Verification items for the finished model (mm, model axes). Round coordinates to 2 decimals unless told otherwise and drop trailing zeros. Loops run counter-clockwise (first coordinate to the right, second up) from the corner with the lowest first, then second, coordinate; pieces in that order, holes last. Notation, with made-up numbers: (-32, 47.5) -> (24, 47.5) arc R17 cw to (24, 51.5) -> close; hole circle Ø3 at (26, 84). An arc over 180 degrees is marked (long way). Write item = value, one per line.
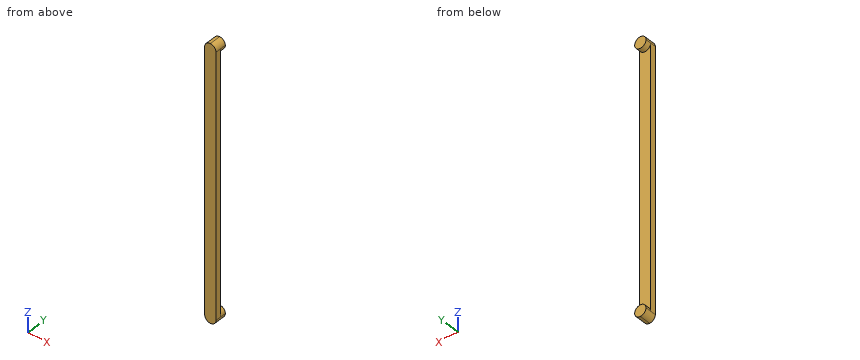
```python
from build123d import *

# Parameters (mm, degrees)
F1_DEPTH = 25.4
F2_DEPTH = 50.8


with BuildPart() as f1:
    # F0 (on Front) → F1 (new body)
    with BuildSketch(Plane.XZ):
        with BuildLine():
            Line((25.4, -584.2), (25.4, 584.2))
            ThreePointArc((25.4, 584.2), (0, 558.8), (-25.4, 584.2))
            Line((-25.4, 584.2), (-25.4, -584.2000000301))
            ThreePointArc((-25.4, -584.2000000301), (-1.51e-08, -558.8), (25.4, -584.2))
        make_face()
    extrude(amount=-F1_DEPTH)

    # F0 (on Front) → F2 (join)
    with BuildSketch(Plane.XZ):
        with BuildLine():
            ThreePointArc((25.4, 584.2), (17.9605121413, 602.160512343), (-2.853e-07, 609.6))
            ThreePointArc((-2.853e-07, 609.6), (-17.960512343, 602.1605121413), (-25.4, 584.2))
            ThreePointArc((-25.4, 584.2), (0, 558.8), (25.4, 584.2))
        make_face()
        with BuildLine():
            ThreePointArc((4.74e-07, -609.6), (17.9605124097, -602.1605120745), (25.4, -584.2))
            ThreePointArc((25.4, -584.2), (-1.51e-08, -558.8), (-25.4, -584.2000000301))
            ThreePointArc((-25.4, -584.2000000301), (-17.9605120639, -602.1605124204), (4.74e-07, -609.6))
        make_face()
    extrude(amount=-F2_DEPTH)


solid = f1.part
```
(1) Sectioned sample at A-A, the plane y = 34.5. Record the cut outline in (x, z).
Filled sheet:
outline = circle Ø50.8 at (0, -584.2); circle Ø50.8 at (0, 584.2)
(2) Sectioned sample at C-C, the plane z = 242.5. Record the cut outline in (x, y).
Filled sheet:
outline = (-25.4, 0) -> (25.4, 0) -> (25.4, 25.4) -> (-25.4, 25.4) -> close
(3) Go/stop test with flat-tipped pins: pin 1 Ø4 at (x, z) = (-20, 467) entering from +Y; pin 2 Ø5 at (x, y) = (12, 35) entering from +Z; pin 3 Ø8 at (x, y) = (-12, 9.5) entering from +Z. Record where each tip stops, or that it passes through.
Filled sheet:
pin_1 = 25.4
pin_2 = 607.76
pin_3 = 608.31
(4) Sectioned sample at B-B, the plane x = 17.5. Record the cut outline in (y, z).
Filled sheet:
outline = (0, -602.61) -> (50.8, -602.61) -> (50.8, -565.79) -> (25.4, -565.79) -> (25.4, 565.79) -> (50.8, 565.79) -> (50.8, 602.61) -> (0, 602.61) -> close
(5) Material ranges on probe 1 along Z at (x, y) = (2.5, 32); probe 2 along Y at (x, z) = (18, 178.5); probe 3 along Z at (x, y) = (7, 34), recorded low to high. Write a range as from..to.
Filled sheet:
probe_1 = -609.48..-558.92, 558.92..609.48
probe_2 = 0..25.4
probe_3 = -608.62..-559.78, 559.78..608.62
